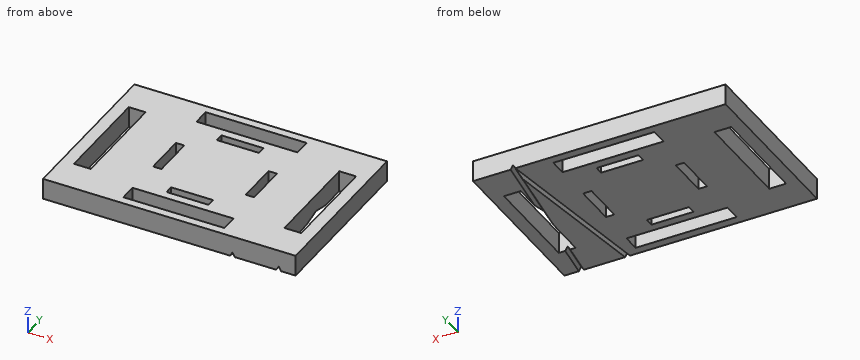
from build123d import *

# Parameters (mm, degrees)
SKETCH_1_W          = 60
SKETCH_1_H          = 40
EXTRUDE_1_DEPTH     = 5
SKETCH_2_W          = 2
SKETCH_2_H          = 10
SKETCH_2_W_2        = 10
SKETCH_2_H_2        = 2
SKETCH_2_W_3        = 4
SKETCH_2_H_3        = 24
SKETCH_2_W_4        = 24
SKETCH_2_H_4        = 4
CUT_EXTRUDE_1_DEPTH = 73.284161474
SWEEP_START         = -34
SWEEP_2_DEPTH       = 43
SWEEP_2_2_DEPTH     = 48


with BuildPart() as part:
    # 草图1 → 凸台-拉伸1 (new body)
    with BuildSketch(Plane.XY):
        with Locations((30, 20)):
            Rectangle(SKETCH_1_W, SKETCH_1_H)
    extrude(amount=EXTRUDE_1_DEPTH)

    # 草图2 → 切除-拉伸1 (cut, through all)
    with BuildSketch(Plane.XY.offset(5)):
        with Locations((19, 20)):
            Rectangle(SKETCH_2_W, SKETCH_2_H)
        with Locations((41, 20)):
            Rectangle(SKETCH_2_W, SKETCH_2_H)
        with Locations((30, 31)):
            Rectangle(SKETCH_2_W_2, SKETCH_2_H_2)
        with Locations((30, 9)):
            Rectangle(SKETCH_2_W_2, SKETCH_2_H_2)
        with Locations((5, 20)):
            Rectangle(SKETCH_2_W_3, SKETCH_2_H_3)
        with Locations((55, 20)):
            Rectangle(SKETCH_2_W_3, SKETCH_2_H_3)
        with Locations((30, 36)):
            Rectangle(SKETCH_2_W_4, SKETCH_2_H_4)
        with Locations((30, 4)):
            Rectangle(SKETCH_2_W_4, SKETCH_2_H_4)
    extrude(amount=-CUT_EXTRUDE_1_DEPTH, mode=Mode.SUBTRACT)

    # 切除-扫描2: read off the stored shape, not the designer's step
    # 切除-扫描2 outline → 切除-扫描2 (cut)
    with BuildSketch(Plane(origin=(0, 0, 0), x_dir=(0.9906788398452959, 0.13621834047872788, 0), z_dir=(0.13621834047872786, -0.9906788398452959, 0)).offset(SWEEP_START)):
        Polygon((56.049983726, 0), (55.478015031, 1), (54.906046336, 0), align=None)
    extrude(amount=SWEEP_2_DEPTH, mode=Mode.SUBTRACT)

    # Sweep 2 2 outline → Sweep 2 2 (cut)
    with BuildSketch(Plane(origin=(0, 0, 0), x_dir=(0.9906788398452959, -0.13621834047872777, 0), z_dir=(0.13621834047872777, 0.9906788398452959, 0))):
        Polygon((45.152516488, 0), (44.008579098, 0), (44.580547793, -1), align=None)
    extrude(amount=SWEEP_2_2_DEPTH, mode=Mode.SUBTRACT)


solid = part.part
Here's how the part is built. I have some questions about the finished solid (model axes, mm). Round coordinates to 2 decimals unless told otherwise and drop trailing zeros. Loops run counter-clockwise (first coordinate to the right, second up) from the corner with the lowest first, then second, coordinate; pieces in that order, holes last.
1. If I drill on line 1 along Y through (x, z) = (23.5, 4.25); line 2 along X through (y, z) = (20.5, 4.7); line 3 along X through (y, z) = (12, 2.85), over which ranges is the centre line in solid material (lowest first)?
Answer list:
line 1: y = 0 to 2, 6 to 34, 38 to 40
line 2: x = 0 to 3, 7 to 18, 20 to 40, 42 to 53, 57 to 60
line 3: x = 0 to 3, 7 to 53, 57 to 60
2. If we section it at C-C on y = 28.5: Write out the boundary of the cut face in (x, z).
Answer list:
outline: (0, 0) - (3, 0) - (3, 5) - (0, 5) - close; (7, 0) - (48.34, 0) - (48.92, 1) - (49.5, 0) - (51.5, 0) - (52.08, 1) - (52.66, 0) - (53, 0) - (53, 5) - (7, 5) - close; (57, 0) - (60, 0) - (60, 5) - (57, 5) - close
3. If we section it at D-D on z = 3.75: Count the separate pieces of the cut face and the enclosed holes in it, plus the area to 3 significant figures.
Answer list:
separate pieces: 1
enclosed holes: 8
area: 1,940 mm2
4. If we section it at A-A on x = 26.5: Write out the boundary of the cut face in (y, z), plus the area to 3 significant figures.
Answer list:
outline: (0, 0) - (2, 0) - (2, 5) - (0, 5) - close; (6, 0) - (8, 0) - (8, 5) - (6, 5) - close; (10, 0) - (30, 0) - (30, 5) - (10, 5) - close; (32, 0) - (34, 0) - (34, 5) - (32, 5) - close; (38, 0) - (40, 0) - (40, 5) - (38, 5) - close
area: 140 mm2
5. If we section it at B-B on y = 3: Write out the boundary of the cut face in (x, z), plus the area to 3 significant figures.
Answer list:
outline: (0, 0) - (18, 0) - (18, 5) - (0, 5) - close; (42, 0) - (44.84, 0) - (45.41, 1) - (45.99, 0) - (55.01, 0) - (55.59, 1) - (56.16, 0) - (60, 0) - (60, 5) - (42, 5) - close
area: 179 mm2
